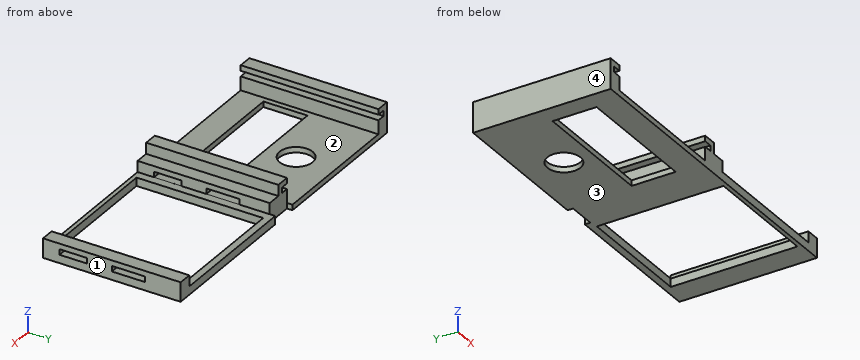
Autodesk Inventor part; units mm, degrees
ref_plane "YZ Plane" through (0, 0, 0) normal (1, 0, 0) x (0, 1, 0)
ref_plane "XZ Plane" through (0, 0, 0) normal (0, 1, 0) x (-1, 0, 0)
ref_plane "XY Plane" through (0, 0, 0) normal (0, 0, 1) x (1, 0, 0)
sketch "Sketch1" plane through (0, 0, 0) normal (0, 0, 1) x (1, 0, 0)
  line L0 (-60, 27.5) -> (-4, 27.5)
  line L1 (-60, -27.5) -> (-60, 27.5)
  line L2 (60, 27.5) -> (60, -27.5)
  line L3 (60, -27.5) -> (-60, -27.5)
  line L4 (10, -17) -> (50, -17)
  line L5 (-10, -13) -> (-10, -3)
  line L6 (-10, -3) -> (-20, -3)
  line L7 (-20, -3) -> (-20, -13)
  line L8 (-20, -13) -> (-10, -13)
  line L9 (60, -27.5) -> (-60, -27.5)
  line L10 (60, 27.5) -> (60, -27.5)
  line L11 (4, 27.5) -> (60, 27.5)
  arc A0 (-4, 27.5) -> (4, 27.5) centre (0, 27.5) ccw
  line L12 (-60, 27.5) -> (-4, 27.5)
  line L13 (-60, -27.5) -> (-60, 27.5)
  circle A1 centre (-30, 10.2208) radius 3
  line L14 (50, 17) -> (10, 17)
  line L15 (50, -17) -> (50, 17)
  line L16 (10, -17) -> (50, -17)
  line L17 (10, 17) -> (10, -17)
  line L18 (-40, -3) -> (-50, -3)
  line L19 (-40, -13) -> (-40, -3)
  line L20 (-50, -13) -> (-40, -13)
  line L21 (-50, -3) -> (-50, -13)
  line L22 (-25, -3) -> (-35, -3)
  line L23 (-25, -13) -> (-25, -3)
  line L24 (-35, -13) -> (-25, -13)
  line L25 (-35, -3) -> (-35, -13)
  line L26 (-10, -3) -> (-20, -3)
  line L27 (-10, -13) -> (-10, -3)
  line L28 (-20, -13) -> (-10, -13)
  line L29 (-20, -3) -> (-20, -13)
  line L30 (-35, -13) -> (-25, -13)
  line L31 (-35, -3) -> (-35, -13)
  circle A2 centre (-30, 10.2208) radius 3
  line L32 (-60, 27.5) -> (60, 27.5)
  line L33 (60, 27.5) -> (60, -27.5)
  line L34 (60, -27.5) -> (-60, -27.5)
  line L35 (-60, -27.5) -> (-60, 27.5)
  line L36 (10, 17) -> (50, 17)
  line L37 (50, 17) -> (50, -17)
  line L38 (50, -17) -> (10, -17)
  line L39 (10, -17) -> (10, 17)
  line L40 (-50, -3) -> (-40, -3)
  line L41 (-40, -3) -> (-40, -13)
  line L42 (-40, -13) -> (-50, -13)
  line L43 (-50, -13) -> (-50, -3)
  line L44 (-35, -3) -> (-25, -3)
  line L45 (-25, -3) -> (-25, -13)
  line L46 (-25, -13) -> (-35, -13)
  line L47 (-35, -13) -> (-35, -3)
  line L48 (-20, -3) -> (-10, -3)
  line L49 (-10, -3) -> (-10, -13)
  line L50 (-10, -13) -> (-20, -13)
  line L51 (-20, -13) -> (-20, -3)
  circle A3 centre (-30, 10.2208) radius 3
  arc A4 (-4, 27.5) -> (4, 27.5) centre (0, 27.5) ccw
  point P0 (0, 0)
  dimension "d0" = 6
extrude "Extrusion1" add sketch "Sketch1" along normal blind 3 contours L0 A0 L11 L2 L3 L1
sketch "Sketch2" plane through (0, 0, 3) normal (0, 0, 1) x (1, 0, 0)
  line L0 (10, 17) -> (50, 17)
  line L1 (8, 22) -> (51, 22)
  line L2 (51, 22) -> (51, -24)
  line L3 (51, -24) -> (8, -24)
  line L4 (8, -24) -> (8, 22)
  line L5 (10, -17) -> (10, 17)
  line L6 (50, -17) -> (10, -17)
  line L7 (50, 17) -> (50, -17)
  circle A0 centre (-30, 10.2208) radius 3
  circle A1 centre (-30, 10.2208) radius 6
  line L8 (-53, 0) -> (-7, 0)
  line L9 (-7, 0) -> (-7, -16)
  line L10 (-7, -16) -> (-53, -16)
  line L11 (-53, -16) -> (-53, 0)
  line L12 (-50, -13) -> (-50, -3)
  line L13 (-40, -13) -> (-50, -13)
  line L14 (-25, -13) -> (-35, -13)
  line L15 (-10, -3) -> (-10, -13)
  line L16 (-10, -13) -> (-20, -13)
  line L17 (-35, -3) -> (-25, -3)
  point P0 (0, 0)
  dimension "d4" = 5
  dimension "d5" = 2
  dimension "d6" = 7
  dimension "d7" = 1
  dimension "d10" = 12
  dimension "d11" = 3
  dimension "d12" = 3
  dimension "d13" = 3
  dimension "d14" = 3
extrude "Extrusion2" cut sketch "Sketch2" against normal blind 3
sketch "Sketch6" plane through (0, 0, 3) normal (0, 0, 1) x (1, 0, 0)
  line L0 (-60, 27.5) -> (-60, -27.5)
  line L1 (-60, -27.5) -> (60, -27.5)
  line L2 (-60, 27.5) -> (-55, 27.5)
  line L3 (-55, 27.5) -> (-55, -27.5)
  line L4 (-55, -27.5) -> (-60, -27.5)
  line L5 (-60, -27.5) -> (-60, 27.5)
  line L6 (-4, 27.5) -> (-60, 27.5)
  line L7 (0, -27.5) -> (-5, -27.5)
  line L8 (-5, -27.5) -> (-5, 27.5)
  line L9 (-5, 27.5) -> (0, 27.5)
  line L10 (0, 27.5) -> (0, -27.5)
  arc A0 (-4, 27.5) -> (4, 27.5) centre (0, 27.5) ccw
  point P0 (0, 0)
  point P1 (0, -27.5)
  point P2 (-5, -27.5)
  point P3 (0, 23.5)
  dimension "d23" = 5
  dimension "d24" = 5
extrude "Extrusion5" add sketch "Sketch6" along normal blind 8 contours L2 L3 L1 L0 | L6 A0 L10 L1 L8 | L9 L10 A0
sketch "Sketch7" plane through (-60, 27.5, 0) normal (0, 1, 0) x (1, 0, 0)
  line L0 (5, -3) -> (5, -11) construction
  line L1 (5, -3) -> (5, -7) construction
  line L2 (5, -7) -> (2, -7)
  line L3 (2, -7) -> (2, -9)
  line L4 (2, -9) -> (5, -9)
  line L5 (55, -3) -> (5, -3)
  line L6 (30, -3) -> (30, -9) construction
  line L7 (55, -3) -> (55, -11) construction
  line L8 (55, -3) -> (55, -7) construction
  line L9 (55, -7) -> (58, -7)
  line L10 (58, -7) -> (58, -9)
  line L11 (58, -9) -> (55, -9)
  line L12 (5, -7) -> (5, -9)
  line L13 (55, -7) -> (55, -9)
  point P0 (60, 0)
  dimension "d27" = 4
  dimension "d28" = 3
  dimension "d29" = 2
extrude "Extrusion6" cut sketch "Sketch7" against normal through all
sketch "Sketch10" plane through (0, 0, 3) normal (0, 0, 1) x (1, 0, 0)
  line L0 (-55, -27.5) -> (-55, 27.5)
  line L1 (-5, 27.5) -> (-5, -27.5)
  line L2 (-55, 27.5) -> (-5, 27.5)
  line L3 (-5, 27.5) -> (-5, -27.5)
  line L4 (-5, -27.5) -> (-55, -27.5)
  line L5 (-55, -27.5) -> (-55, 27.5)
  point P0 (0, 0)
extrude "Extrusion9" cut sketch "Sketch10" against normal blind 1
sketch "Sketch11" plane through (0, 0, 3) normal (0, 0, 1) x (1, 0, 0)
  line L0 (0, -27.5) -> (0, 27.5)
  line L1 (-60, -27.5) -> (60, -27.5)
  line L2 (0, 27.5) -> (5, 27.5)
  line L3 (5, 27.5) -> (5, -27.5)
  line L4 (5, -27.5) -> (0, -27.5)
  line L5 (0, -27.5) -> (0, 27.5)
  line L6 (60, -27.5) -> (60, 27.5)
  line L7 (60, 27.5) -> (55, 27.5)
  line L8 (55, 27.5) -> (55, -27.5)
  line L9 (55, -27.5) -> (60, -27.5)
  line L10 (60, -27.5) -> (60, 27.5)
  point P0 (0, 0)
  dimension "d43" = 5
  dimension "d44" = 5
extrude "Extrusion10" add sketch "Sketch11" along normal blind 4
sketch "Sketch14" plane through (60, -27.5, 0) normal (1, 0, 0) x (0, 0, -1)
  point P0 (0, 27.5)
sketch "Sketch15" plane through (60, -27.5, 0) normal (1, 0, 0) x (0, 0, -1)
  line L0 (-2, 55) -> (-2, 0)
  line L1 (-7, 0) -> (-2, 0)
  line L2 (-3.0003, 0.0005) -> (-3.0003, 18)
  line L3 (-2, 0) -> (-2, 55)
  line L4 (-3.0003, 18) -> (-5.0003, 18)
  line L5 (-5.0003, 18) -> (-5.0003, 8)
  line L6 (-5.0003, 8) -> (-3.0003, 8)
  line L7 (-2.9987, 54.9727) -> (-2.9987, 27)
  line L8 (-2.9987, 27) -> (-5.0003, 27)
  line L9 (-5.0003, 27) -> (-5.0003, 39)
  line L10 (-5.0003, 39) -> (-2.9987, 39)
  line L11 (-3, 0) -> (-3, 55)
  line L12 (0, 55) -> (-7, 55)
  point P0 (0, 27.5)
  point P1 (-2, 39)
  point P2 (-2, 8)
  point P3 (-2, 18)
  dimension "d65" = 2
  dimension "d66" = 10
  dimension "d68" = 12
  dimension "d71" = 28
  dimension "d72" = 18
extrude "Extrusion13" cut sketch "Sketch15" against normal up to surface (60 mm away) contours L6 L5 L4 L2 | L7 L8 L9 L10
sketch "Sketch16" plane through (0, 0, 11) normal (0, 0, 1) x (1, 0, 0)
  line L0 (-60, 27.5) -> (-60, -27.5)
  line L1 (60, -27.5) -> (60, 27.5)
  line L2 (-60, 27.5) -> (60, 27.5)
  line L3 (60, 27.5) -> (60, 24.5)
  line L4 (60, 24.5) -> (-60, 24.5)
  line L5 (-60, 24.5) -> (-60, 27.5)
  line L6 (-60, -27.5) -> (60, -27.5)
  line L7 (-60, -27.5) -> (60, -27.5)
  line L8 (60, -27.5) -> (60, -25.5)
  line L9 (60, -25.5) -> (-60, -25.5)
  line L10 (-60, -25.5) -> (-60, -27.5)
  line L11 (-55, 27.5) -> (-5, 27.5)
  line L12 (5, 27.5) -> (5, 11.5)
  line L13 (-5, 27.5) -> (5, 27.5)
  line L14 (5, 27.5) -> (5, 24.5)
  line L15 (5, 24.5) -> (-5, 24.5)
  line L16 (-5, 24.5) -> (-5, 27.5)
  line L17 (-5, 24.5) -> (5, 24.5)
  line L18 (5, 24.5) -> (5, 22.5)
  line L19 (5, 22.5) -> (-5, 22.5)
  line L20 (-5, 22.5) -> (-5, 24.5)
  point P0 (0, 0)
  point P1 (-60, -25.5)
  dimension "d74" = 3
  dimension "d77" = 2
  dimension "d78" = 2
extrude "Extrusion14" cut sketch "Sketch16" against normal through all contours L2 L16 L4 L0 | L9 L1 L6 L0 | L16 L2 L12 L4 | L4 L12 L19 L20 | L12 L2 L1 L4
properties part number "circuit clip_3DPrint"
Source: CAD feature listing. Evaluate the final solid. Frame: model axes, mm. Face numbers are marked on the shaded views. Coordinates: 2 decimals unless noted, no trailing zeros. Loops run counter-clockwise (first coordinate to the right, second up) from the corner with the lowest first, then second, coordinate; pieces in that order, holes last. Notation, with made-up numbers: M -28,82.5 L -21,82.5 A19 cw -21,103.5 Z; hole C 80,-1 d6. An arc over 180 degrees is marked long. Put each result on its own line as item: value. Start each with the question number.
1) Cut plane C-C on x = 12. Return the cut outline in (y, z), then the cut area to 3 significant figures.
2) Contact query for flat-ended pins moving along their axis: pin 1 Ø3 at (y, z) = (5.5, 3.5) entering from +X; pin 2 Ø1 at (x, z) = (2, 4) entering from +Y; pin 3 Ø6 at (x, y) = (-11, -2) entering from +Z; pin 4 Ø1.5 at (y, z) = (3.5, 4) entering from +X. Output: stop coordinate, or through.
3) Pull-direction query (X, two-part tool) for the marked faces 1, 2, 3 and 4; classes: pulls with the +X half, pulls with the -X half, needs draft (parallel to the pull), parting line crosses it, or undercut.
4) Cut plane B-B on y = -7. Give the number of separate pieces and of enclosed holes in the cut face, then the cut area to 3 significant figures.
5) Cut plane A-A on x = -30. Return the cut outline in (y, z).
6) Ray query, L1, parallel to X at y = -5, z = 6; L2, parallel to Y at x = -30, z = 1.3; L3, parallel to X at y = 2, z = 4.75. Return the intervals inside material, ascending. Write a range as from..to.
7) Cut plane D-D on x = -14.5. Return the cut outline in (y, z).
The answers:
1. outline: M -25.5,0 L -24,0 L -24,3 L -25.5,3 Z; M 22,0 L 24.5,0 L 24.5,3 L 22,3 Z
1. area: 12.0 mm²
2. pin 1: stops at x = 60
2. pin 2: stops at y = 22.5
2. pin 3: stops at z = 2
2. pin 4: stops at x = 0
3. face 1: pulls with the +X half
3. face 2: undercut
3. face 3: needs draft
3. face 4: pulls with the -X half
4. separate pieces: 3
4. enclosed holes: 0
4. area: 197 mm²
5. outline: M -25.5,0 L -16,0 L -16,2 L -25.5,2 Z; M 0,0 L 4.22,0 L 4.22,2 L 0,2 Z; M 16.22,0 L 24.5,0 L 24.5,2 L 16.22,2 Z
6. L1: x = -60..-55, -5..5, 55..60
6. L2: y = -25.5..-16, 0..4.22, 16.22..24.5
6. L3: x = -60..-55, -5..0
7. outline: M -25.5,0 L -16,0 L -16,2 L -25.5,2 Z; M 0,0 L 24.5,0 L 24.5,2 L 0,2 Z
